Solid Edge part; units mm, degrees
sketch "Sketch1" plane through (0, 0, 0) normal (0, -1, 0) x (1, 0, 0)
  circle A0 centre (0, 0) radius 6.65
extrude "Protrusion1" add sketch "Sketch1" along normal blind 46.87
sketch "Sketch2" plane through (0, -46.87, 0) normal (0, -1, 0) x (1, 0, 0)
  line L0 (-4.1, 4.1) -> (4.1, 4.1)
  line L1 (4.1, 4.1) -> (4.1, -4.1)
  line L2 (4.1, -4.1) -> (-4.1, -4.1)
  line L3 (-4.1, -4.1) -> (-4.1, 4.1)
  dimension "D1" = 4.1
extrude "Cutout1" cut sketch "Sketch2" against normal through all
sketch "Sketch3" plane through (0, -46.87, 0) normal (0, -1, 0) x (1, 0, 0)
  line L0 (4.1, -4.1) -> (-4.1, -4.1)
  line L1 (-4.1, -4.1) -> (-4.1, 4.1)
  line L2 (-4.1, 4.1) -> (4.1, 4.1)
  line L3 (4.1, 4.1) -> (4.1, -4.1)
  line L4 (-4.5826, 10) -> (4.5826, 10)
  arc A0 (4.5826, 10) -> (10, 4.5826) centre (0, 0) cw
  line L5 (10, 4.5826) -> (10, -4.5826)
  line L6 (-4.5826, -10) -> (4.5826, -10)
  arc A1 (-4.5826, -10) -> (-10, -4.5826) centre (0, 0) cw
  line L7 (-10, 4.5826) -> (-10, -4.5826)
  arc A2 (-10, 4.5826) -> (-4.5826, 10) centre (0, 0) cw
  arc A3 (10, -4.5826) -> (4.5826, -10) centre (0, 0) cw
extrude "Protrusion2" add sketch "Sketch3" against normal up to vertex (5.5 mm away)
sketch "Sketch4" plane through (0, -42.25, 8.7) normal (0, 0, 1) x (1, 0, 0)
  line L0 (-2.85, 0.88) -> (2.85, 0.88)
  line L1 (2.85, 0.88) -> (2.85, -4.62)
  line L2 (2.85, -4.62) -> (-2.85, -4.62)
  line L3 (-2.85, -4.62) -> (-2.85, 0.88)
extrude "Extrusionsausschnitt_2" cut sketch "Sketch4" against normal blind 2
hole "Hole1" at (0, -44.12, 10) direction (0, 0, -1) diameter 3.5 end through all
pattern_circular "Pattern1" count 4 over 360 about axis through (0, -46.87, 0) along (0, -1, 0) of "Hole1", "Extrusionsausschnitt_2"
Read the model definition and answer for the solid it produces. Units are mm, in the model's axes. A direction names the side the tool comes from. Round coordinates to 2 decimals unless told otherwise and drop trailing zeros. Order: outer loops, then holes, each group sorted by start corner. A loop starts at its lowest first (then second) coordinate and runs counter-clockwise, first axis right, second up. Notation, with made-up numbers: (66, 52) - (79, 52) arc R11 cw to (79, 58) - close; hole circle Ø1 at (51, 54.5). An arc over 180 degrees is marked (long way). Use one line per item in the form item = value. Start each with the question number.
(1) Flat-ended cylindrical pins translate along their axes: pin 1 Ø4.5 at (x, y) = (1.5, -43.5) entering from -Z; pin 2 Ø1.5 at (y, z) = (-24.5, -3) entering from -X; pin 3 Ø1 at (x, y) = (6.5, -5) entering from -Z; pin 4 Ø4 at (x, y) = (-2, -16) entering from +Z. Find the tip coordinate at first contact, or state that the pin passes through.
(2) The part is cut by section C-C (x = 0). Count the separate pieces of the cut face and the enclosed holes in it, then the cut area to 3 significant figures.
(3) The part is cut by section A-A (y = -23). Give the vertices of the cut face in (x, z).
(4) The part is cut by section B-B (z = -2.25). Give the vertices of the cut face in (x, y).
(5) Determine the mould class of faces 1 (the face through (-8, -44, -2.85)), 2 (the face through (9.341, -45.737, -0.67)), 3 (the face through (-2.85, -44, 8)), 4 (the face through (-7.739, -44.158, 7.817)) for opening direction X: +X half, -X half, draft (parallel to the pull), parting line (faces both ways), or undercut.
(6) Find the intervals of material crossed by line 1 along X through (y, z) = (-41.5, -1); line 2 along Y through (x, z) = (-5.8, 0); line 3 along Y through (x, z) = (-5.5, -0.5), in increasing order. Write a range as from..to.
(7) For faces 5 (the face through (3.07, -20.4, 5.9)), 6 (the face through (0.1, 0, -4.3)), 7 (the face through (8.7, -42, 0)), determine the directions among +Z, -Z, +X, -X, +Y, -Y from which every point of the face is accessible in a straight line to the end or side of a thin tool.
(8) The part is cut by section D-D (z = 5.5). Give the vertices of the cut face in (x, y), then the cut area to 3 significant figures.
Checked values:
q1.pin_1 = -10
q1.pin_2 = -6.26
q1.pin_3 = -2.87
q1.pin_4 = 6.65
q2.separate_pieces = 8
q2.enclosed_holes = 0
q2.area = 227 mm^2
q3.outline = circle Ø13.3 at (0, 0); hole (-4.1, -4.1) - (4.1, -4.1) - (4.1, 4.1) - (-4.1, 4.1) - close
q4.outline = (-10, -46.87) - (-8.7, -46.87) - (-8.7, -41.37) - (-10, -41.37) - close; (-6.7, -46.87) - (-4.1, -46.87) - (-4.1, 0) - (-6.26, 0) - (-6.26, -41.37) - (-6.7, -41.37) - close; (4.1, -46.87) - (6.7, -46.87) - (6.7, -41.37) - (6.26, -41.37) - (6.26, 0) - (4.1, 0) - close; (8.7, -46.87) - (10, -46.87) - (10, -41.37) - (8.7, -41.37) - close
q5.face_1 = undercut
q5.face_2 = draft
q5.face_3 = undercut
q5.face_4 = -X half
q6.line_1 = -10..-8.7, -6.7..-4.1, 4.1..6.7, 8.7..10
q6.line_2 = -46.87..-45.87, -42.37..0
q6.line_3 = -46.87..-45.8, -42.44..0
q7.face_5 = +Y
q7.face_6 = +Z, -Z, +X, -X, +Y
q7.face_7 = +Y, -Y
q8.outline = (-9.53, -46.87) - (9.53, -46.87) - (9.53, -41.37) - (3.74, -41.37) - (3.74, 0) - (-3.74, 0) - (-3.74, -41.37) - (-9.53, -41.37) - close; hole circle Ø3.5 at (0, -44.12)
q8.area = 404 mm^2
